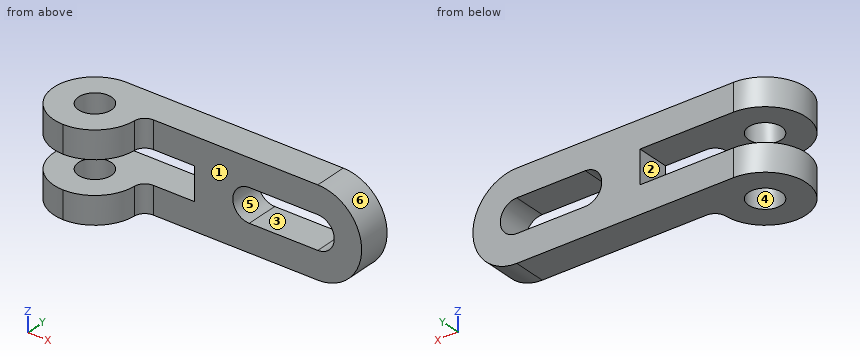
from build123d import *

# Parameters (mm, degrees)
F1_DEPTH = 12
F2_DEPTH = 30
F3_DEPTH = 25
F4_DEPTH = 25
F5_R     = 6
F5_W     = 16
F5_H     = 12
F6_DEPTH = 46.7


with BuildPart() as f1:
    # F0 (on Front) → F1 (new body)
    with BuildSketch(Plane.XZ):
        with BuildLine():
            Line((-94, -16), (0, -16))
            ThreePointArc((0, -16), (16, 0), (0, 16))
            Line((0, 16), (-94, 16))
            Line((-94, 16), (-94, 6))
            Line((-94, 6), (-45, 6))
            Line((-45, 6), (-45, -6))
            Line((-45, -6), (-94, -6))
            Line((-94, -6), (-94, -16))
        make_face()
        with BuildLine():
            ThreePointArc((-25, -6), (-31, 0), (-25, 6))
            Line((-25, 6), (0, 6))
            ThreePointArc((0, 6), (6, 0), (0, -6))
            Line((0, -6), (-25, -6))
        make_face(mode=Mode.SUBTRACT)
        with BuildLine():
            Line((0, 6), (-25, 6))
            ThreePointArc((-25, 6), (-31, 0), (-25, -6))
            Line((-25, -6), (0, -6))
            ThreePointArc((0, -6), (6, 0), (0, 6))
        make_face()
    extrude(amount=F1_DEPTH)

    # F0 (on Front) → F2 (join)
    with BuildSketch(Plane.XZ):
        with BuildLine():
            Line((-94, -16), (0, -16))
            ThreePointArc((0, -16), (16, 0), (0, 16))
            Line((0, 16), (-94, 16))
            Line((-94, 16), (-94, 6))
            Line((-94, 6), (-45, 6))
            Line((-45, 6), (-45, -6))
            Line((-45, -6), (-94, -6))
            Line((-94, -6), (-94, -16))
        make_face()
        with BuildLine():
            ThreePointArc((-25, -6), (-31, 0), (-25, 6))
            Line((-25, 6), (0, 6))
            ThreePointArc((0, 6), (6, 0), (0, -6))
            Line((0, -6), (-25, -6))
        make_face(mode=Mode.SUBTRACT)
    extrude(amount=F2_DEPTH)

    # F0 (on Front) → F3 (join)
    with BuildSketch(Plane.XZ):
        with BuildLine():
            Line((0, 6), (-25, 6))
            ThreePointArc((-25, 6), (-31, 0), (-25, -6))
            Line((-25, -6), (0, -6))
            ThreePointArc((0, -6), (6, 0), (0, 6))
        make_face()
    extrude(amount=F3_DEPTH)

    # F0 (on Front) → F4 (cut)
    with BuildSketch(Plane.XZ):
        with BuildLine():
            Line((0, 6), (-25, 6))
            ThreePointArc((-25, 6), (-31, 0), (-25, -6))
            Line((-25, -6), (0, -6))
            ThreePointArc((0, -6), (6, 0), (0, 6))
        make_face()
    extrude(amount=F4_DEPTH, mode=Mode.SUBTRACT)

    # F5 (on face) → F6 (intersect)
    with BuildSketch(Plane.XY.offset(16)):
        with BuildLine():
            Line((0, 0), (-79, 0))
            ThreePointArc((-79, 0), (-89.6066017178, -4.3933982822), (-94, -15))
            ThreePointArc((-94, -15), (-89.6066017178, -25.6066017178), (-79, -30))
            ThreePointArc((-79, -30), (-68.6762919758, -25.8821437517), (-64.0207900308, -15.7894736842))
            ThreePointArc((-64.0207900308, -15.7894736842), (-62.7793228454, -13.0980949996), (-60.026334039, -12))
            Line((-60.026334039, -12), (0, -12))
            Line((0, -12), (0, 0))
        make_face()
        with Locations((-79, -15)):
            Circle(F5_R, mode=Mode.SUBTRACT)
        with Locations((8, -6)):
            Rectangle(F5_W, F5_H)
    extrude(amount=-F6_DEPTH, mode=Mode.INTERSECT)


solid = f1.part
Read the model definition and answer for the solid it produces. Units are mm, in the model's axes. Face numbers are marked on the shaded views. A direction names the side the tool comes from. Coordinates: 2 decimals unless noted, no trailing zeros. Order: outer loops, then holes, each group sorted by start corner. A loop starts at its lowest first (then second) coordinate and runs counter-clockwise, first axis right, second up. Notation, with made-up numbers: M -13,-39.5 L 42,-39.5 A21 cw 42,-9.5 Z; hole C 34,16.25 d8. An arc over 180 degrees is marked long. Put each result on its own line as item: value. Start each with the question number.
Item 1: Section C-C, the plane y = -20 is taken. Determine the outline of the cut face in (x, z).
Item 2: Section B-B, the plane z = 0 is taken. Determine the outline of the cut face in (x, y), plus the area to 3 significant figures.
Item 3: The mould has two halves that part along Z. Classify the marked faces 4, 5 and 6: +Z half, -Z half, draft (parallel to the pull), parting line (faces both ways), or undercut.
Item 4: Consider probe 1 along Y at (x, z) = (-79, -13); probe 2 along X at (y, z) = (-9.5, -0.5); probe 3 along Z at (x, y) = (-70.5, -9.25). Determine where each line is inside the solid, lowest interval first. Write a range as [from, to].
Item 5: Given pin 1 Ø8 at (y, z) = (-9.5, 12) entering from +X; pin 2 Ø16 at (x, z) = (-24, 2) entering from -Y; pin 3 Ø1.5 at (y, z) = (-7.5, -4.5) entering from -X, each flat-ended and moving along its own axis, determine where each tip first touches the part or whether it passes through.
Item 6: For the marked faces 1, 2 and 3, determine the directions among +Z, -Z, +X, -X, +Y, -Y from which every point of the face is accessible in a straight line to the end or side of a thin tool.
Item 7: Section A-A, the plane x = -2 is taken. Determine the outline of the cut face in (y, z), plus the area to 3 significant figures.
Item 8: Section D-D, the plane y = -5.5 is taken. Determine the outline of the cut face in (x, z).
Computed:
1. outline: M -93.14,-16 L -82.32,-16 L -82.32,-6 L -93.14,-6 Z; M -93.14,6 L -82.32,6 L -82.32,16 L -93.14,16 Z; M -75.68,-16 L -64.86,-16 L -64.86,-6 L -75.68,-6 Z; M -75.68,6 L -64.86,6 L -64.86,16 L -75.68,16 Z
2. outline: M -45,-12 L -31,-12 L -31,0 L -45,0 Z; M 6,-12 L 16,-12 L 16,0 L 6,0 Z
2. area: 288 mm2
3. face 4: draft
3. face 5: undercut
3. face 6: parting line
4. probe 1: y = [-30, -21], [-9, 0]
4. probe 2: x = [-45, -30.98], [5.98, 15.99]
4. probe 3: z = [-16, -6], [6, 16]
5. pin 1: stops at x = 13.86
5. pin 2: stops at y = -12
5. pin 3: stops at x = -45
6. face 1: +Z, -Z, +X, -Y
6. face 2: -X, +Y, -Y
6. face 3: +Y, -Y
7. outline: M -12,-16 L 0,-16 L 0,-6 L -12,-6 Z; M -12,6 L 0,6 L 0,16 L -12,16 Z
7. area: 240 mm2
8. outline: M -90.61,-16 L 0,-16 A16 ccw 0,16 L -90.61,16 L -90.61,6 L -45,6 L -45,-6 L -90.61,-6 Z; hole M -25,-6 L 0,-6 A6 ccw 0,6 L -25,6 A6 ccw Z
